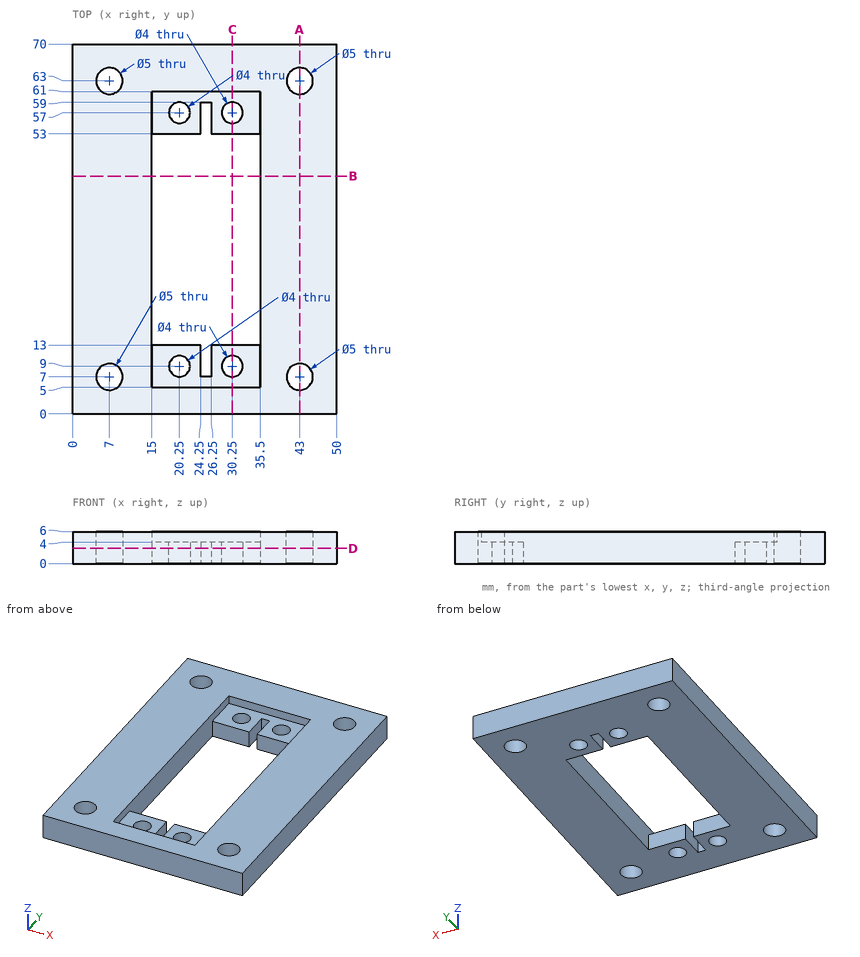
For this review, use the dimensioned drawing (mm, ordinates from the lowest corner) and the shaded views. Coordinates: 2 decimals unless noted, no trailing zeros. Order: outer loops, then holes, each group sorted by start corner. A loop starts at its lowest first (then second) coordinate and runs counter-clockwise, first axis right, second up. Notation, with made-up numbers: (48, 27) - (52, 27) arc R12 ccw to (52, 42) - close; hole circle Ø2 at (77, -17.5). An arc over 180 degrees is marked (long way). Answer in a Markdown table with one row per item.
(1) Consider section C-C on x = 30.25. State the section outline as (y, z) points.
Checked values:
| item | result |
|---|---|
| outline | (0, 0) - (7, 0) - (7, 4) - (5, 4) - (5, 6) - (0, 6) - close; (11, 0) - (13, 0) - (13, 4) - (11, 4) - close; (53, 0) - (55, 0) - (55, 4) - (53, 4) - close; (59, 0) - (70, 0) - (70, 6) - (61, 6) - (61, 4) - (59, 4) - close |
(2) Consider section A-A on x = 43. State the section outline as (y, z) points, plus the area to 3 significant figures.
Checked values:
| item | result |
|---|---|
| outline | (0, 0) - (4.5, 0) - (4.5, 6) - (0, 6) - close; (9.5, 0) - (60.5, 0) - (60.5, 6) - (9.5, 6) - close; (65.5, 0) - (70, 0) - (70, 6) - (65.5, 6) - close |
| area | 360 mm^2 |
(3) Consider section B-B on y = 45. State the section outline as (x, z) points, plus the area to 3 significant figures.
Checked values:
| item | result |
|---|---|
| outline | (0, 0) - (15, 0) - (15, 6) - (0, 6) - close; (35.5, 0) - (50, 0) - (50, 6) - (35.5, 6) - close |
| area | 177 mm^2 |
(4) Clearance check with flat-ended pins moving along their axes: pin 1 (3 mm diameter, centred on y = 20.5, z = 2, fed in from -X); pin 2 (2.5 mm diameter, centred on x = 23, y = 56.5, fed in from +Z). State where each tip first meets the part, or that it passes through.
Checked values:
| item | result |
|---|---|
| pin 1 | x = 0 |
| pin 2 | z = 4 |
(5) Consider section D-D on z = 2.85. Give the number of separate pieces and of enclosed holes in the cut face, plus the area to 3 significant figures.
Checked values:
| item | result |
|---|---|
| separate pieces | 1 |
| enclosed holes | 9 |
| area | 2,530 mm^2 |
(6) Wall thickness on line 1 along Y through (x, z) = (20.25, 1.8); line 2 along Y through (x, z) = (7, 3.6); line 3 along X through (y, z) = (43.5, 1): over which ranges is each line inside the solid? List them lowest first. Write a range as from..to.
Checked values:
| item | result |
|---|---|
| line 1 | 0..7, 11..13, 53..55, 59..70 |
| line 2 | 0..4.5, 9.5..60.5, 65.5..70 |
| line 3 | 0..15, 35.5..50 |
